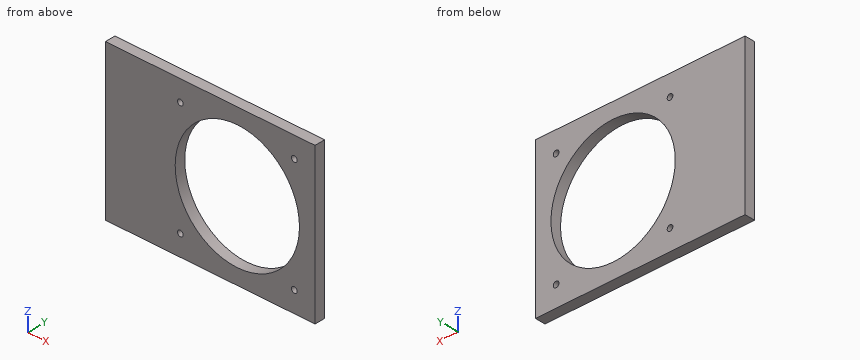
from build123d import *

# Parameters (mm, degrees)
SKETCH5_W           = 128.500510093
SKETCH5_H           = 6.35
BOSS_EXTRUDE1_DEPTH = 95.25
SKETCH6_R           = 38.1
SKETCH6_R_2         = 1.75
CUT_EXTRUDE3_DEPTH  = 7.35


with BuildPart() as part:
    # Sketch5 → Boss-Extrude1 (new body)
    with BuildSketch(Plane.XY):
        with Locations((91.472352703, 307.975)):
            Rectangle(SKETCH5_W, SKETCH5_H)
    extrude(amount=BOSS_EXTRUDE1_DEPTH)

    # Sketch6 → Cut-Extrude3 (cut, through all)
    with BuildSketch(Plane(origin=(0, 311.15, 0), x_dir=(1, 0, 0), z_dir=(0, 1, 0))):
        with Locations((108.097607749, -47.625)):
            Circle(SKETCH6_R)
        with Locations((73.172607749, -12.7)):
            Circle(SKETCH6_R_2)
        with Locations((73.172607749, -82.55)):
            Circle(SKETCH6_R_2)
        with Locations((143.022607749, -82.55)):
            Circle(SKETCH6_R_2)
        with Locations((143.022607749, -12.7)):
            Circle(SKETCH6_R_2)
    extrude(amount=-CUT_EXTRUDE3_DEPTH, mode=Mode.SUBTRACT)


solid = part.part
Design review of the part built by this model. Coordinates are the model's own, in mm. Round coordinates to 2 decimals unless told otherwise and drop trailing zeros. Order: outer loops, then holes, each group sorted by start corner. A loop starts at its lowest first (then second) coordinate and runs counter-clockwise, first axis right, second up. Notation, with made-up numbers: M 59,27.25 L 90,27.25 A33 ccw 90,61.25 Z; hole C 88.25,63 d7. An arc over 180 degrees is marked long. Answer as CSV lines item,"result". Start each with the question number.
1) For pin 1 Ø3 at (x, z) = (143.02, 82.55) entering from -Y, flat-tipped, find the tip position at first contact; note if it passes through.
2) Add section D-D (z = 12.7). Give the boundary of the cut face in (x, y), then the cut area to 3 significant figures.
3) Add section A-A (z = 72). Give the boundary of the cut face in (x, y), then the cut area to 3 significant figures.
4) Wall thickness on line 1 along X through (y, z) = (309, 46.5); line 2 along X through (y, z) = (306.75, 82.55); line 3 along X through (y, z) = (305.5, 28.5): over which ranges is each line inside the solid? List them lowest first. Write a range as [from, to].
5) Add section B-B (x = 102). Give the boundary of the cut face in (y, z).
6) Add section C-C (y = 307.25). Give the boundary of the cut face in (x, z) (3 decimals).
Resolved:
1,pin 1,"through"
2,outline,"M 27.22,304.8 L 71.42,304.8 L 71.42,311.15 L 27.22,311.15 Z; M 74.92,304.8 L 92.87,304.8 L 92.87,311.15 L 74.92,311.15 Z; M 123.32,304.8 L 141.27,304.8 L 141.27,311.15 L 123.32,311.15 Z; M 144.77,304.8 L 155.72,304.8 L 155.72,311.15 L 144.77,311.15 Z"
2,area,"578 mm^2"
3,outline,"M 27.22,304.8 L 78.82,304.8 L 78.82,311.15 L 27.22,311.15 Z; M 137.38,304.8 L 155.72,304.8 L 155.72,311.15 L 137.38,311.15 Z"
3,area,"444 mm^2"
4,line 1,"[27.22, 70.01], [146.18, 155.72]"
4,line 2,"[27.22, 71.42], [74.92, 92.87], [123.32, 141.27], [144.77, 155.72]"
4,line 3,"[27.22, 75.15], [141.05, 155.72]"
5,outline,"M 304.8,0 L 311.15,0 L 311.15,10.02 L 304.8,10.02 Z; M 304.8,85.23 L 311.15,85.23 L 311.15,95.25 L 304.8,95.25 Z"
6,outline,"M 27.222,0 L 155.723,0 L 155.723,95.25 L 27.222,95.25 Z; hole C 108.098,47.625 d76.2; hole C 73.173,12.7 d3.5; hole C 73.173,82.55 d3.5; hole C 143.023,12.7 d3.5; hole C 143.023,82.55 d3.5"
